Could you check a few things on this model? Use its own coordinates, in mm. Face numbers are marked on the shaded views. Round coordinates to 2 decimals unless told otherwise and drop trailing zeros. Write each loop counter-clockwise with the first axis right and the second up, starting at its lowest first coordinate (ties: lowest second). Pieces come first, ordered by that corner, then holes. Notation, with made-up numbers: (43.25, 69) -> (101.25, 69) arc R15 cw to (101.25, 85) -> close; hole circle Ø10 at (73, -16.5). An arc over 180 degrees is marked (long way). Answer in a Markdown table with one row per item. Add a question column.
```python
from build123d import *

# Parameters (mm, degrees)
SKETCH1_R           = 1.5025
BOSS_EXTRUDE1_DEPTH = 3.25


with BuildPart() as part:
    # Sketch1 → Boss-Extrude1 (new body)
    with BuildSketch(Plane(origin=(0, 0, 0), x_dir=(1, 0, 0), z_dir=(0, 1, 0))):
        with BuildLine():
            Line((-14.5, 4), (14.5, 4))
            ThreePointArc((14.5, 4), (17.328427125, 2.828427125), (18.5, 0))
            Line((18.5, 0), (18.5, -4))
            Line((18.5, -4), (-18.5, -4))
            Line((-18.5, -4), (-18.5, 0))
            ThreePointArc((-18.5, 0), (-17.328427125, 2.828427125), (-14.5, 4))
        make_face()
        with Locations((-5, 0.5)):
            Circle(SKETCH1_R, mode=Mode.SUBTRACT)
        with Locations((5, 0.5)):
            Circle(SKETCH1_R, mode=Mode.SUBTRACT)
    extrude(amount=BOSS_EXTRUDE1_DEPTH)


solid = part.part
```
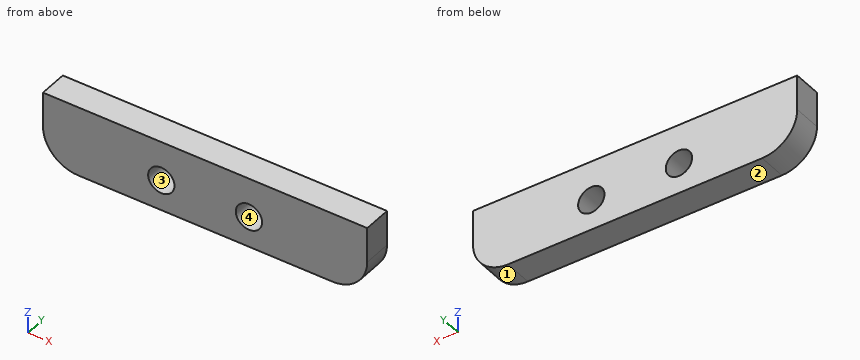
(1) Suppose I cut it at A-A, the plane x = 5. Please give me the cut outline in (y, z), then the cut area to 3 significant figures.
(2) Suppose I cut it at C-C, the plane z = 0.5. Please give me the cut outline in (x, y).
(3) Suppose I cut it at B-B, the plane y = 1.25. Please give me the cut outline in (x, z) (1 decimal).
(4) I need wall thicknesses on L1, parallel to Z at x = 5, y = 0.8; L2, parallel to X at y = 1.6, z = -0.5; L3, parallel to X at y = 0.7, z = 0.5. Which ranges of each line are inside material? Lowest first, please.
(5) If we mould it in two halves opening along X, with no side actions, what happens to the marked faces 1, 2, 3 and 4? For each: pulls with the +X half, pulls with the -X half, needs draft (parallel to the pull), parting line crosses it, or undercut.
(6) Suppose I cut it at D-D, the plane z = -3.25. Please give me the cut outline in (x, y), then the cut area to 3 significant figures.
Response:
| question | item | result |
|---|---|---|
| 1 | outline | (0, -4) -> (3.25, -4) -> (3.25, -2) -> (0, -2) -> close; (0, 1) -> (3.25, 1) -> (3.25, 4) -> (0, 4) -> close |
| 1 | area | 16.2 mm² |
| 2 | outline | (-18.5, 0) -> (-6.12, 0) -> (-6.12, 3.25) -> (-18.5, 3.25) -> close; (-3.88, 0) -> (3.88, 0) -> (3.88, 3.25) -> (-3.88, 3.25) -> close; (6.12, 0) -> (18.5, 0) -> (18.5, 3.25) -> (6.12, 3.25) -> close |
| 3 | outline | (-18.5, 0) arc R4 ccw to (-14.5, -4) -> (14.5, -4) arc R4 ccw to (18.5, 0) -> (18.5, 4) -> (-18.5, 4) -> close; hole circle Ø3 at (-5, -0.5); hole circle Ø3 at (5, -0.5) |
| 4 | L1 | -4 to -2, 1 to 4 |
| 4 | L2 | -18.47 to -6.5, -3.5 to 3.5, 6.5 to 18.47 |
| 4 | L3 | -18.5 to -6.12, -3.88 to 3.88, 6.12 to 18.5 |
| 5 | face 1 | pulls with the +X half |
| 5 | face 2 | needs draft |
| 5 | face 3 | undercut |
| 5 | face 4 | undercut |
| 6 | outline | (-16.83, 0) -> (16.83, 0) -> (16.83, 3.25) -> (-16.83, 3.25) -> close |
| 6 | area | 109 mm² |
